Could you check a few things on this model? Use its own coordinates, in mm. A direction names the side the tool comes from. Round coordinates to 2 decimals unless told otherwise and drop trailing zeros. Order: outer loops, then holes, each group sorted by start corner. A loop starts at its lowest first (then second) coordinate and runs counter-clockwise, first axis right, second up. Notation, with made-up numbers: (27.5, 40) - (54.5, 40) arc R16 cw to (54.5, 54) - close; hole circle Ø5 at (-31, -13). An arc over 180 degrees is marked (long way). Use one line per item in the form item = value.
from build123d import *

# Parameters (mm, degrees)
F2_R             = 8.25
F3_DEPTH         = 3
F4_R             = 8.55
F5_DEPTH         = 17.2
F7_S5_R          = 8.25
F7_T6_DEPTH      = 14
F6_R             = 6.25
F8_DEPTH         = 4
F10_D            = 10.3
F10_DEPTH        = 25
F10_TIP          = 3.094432188
F11_R            = 0.5
F12_SIZE         = 0.5
F14_DEPTH        = 8
F14_COPIES_COUNT = 2


# Not quite as in the source:
# - a fillet or chamfer that OpenCascade refuses, or shapes differently, is made with other operations: its cross-section is extruded or revolved along the edge and cut away or added
# - a pattern or mirror of a feature is missing from the dataset's text; its kind, count and spacing are read off the source's solid


with BuildPart() as f1:
    # F0 (on Right) → F1 (revolve)
    with BuildSketch(Plane.YZ):
        Polygon((0, 25), (0, 0), (57.36, 0), (57.36, 8.9099957178), (9.6, 15.875), (9.6, 15.375), (8, 15.375), (8, 15.875), (8, 25), align=None)
    revolve(axis=Axis((0, 28.68, 0), (0, 1, 0)))

    # F2 (on face) → F3 (join)
    with BuildSketch(Plane(origin=(0, 57.36, 0), x_dir=(-1, 0, 0), z_dir=(0, 1, 0))):
        Circle(F2_R)
    extrude(amount=F3_DEPTH)

    # F4 (on face) → F5 (join)
    with BuildSketch(Plane(origin=(0, 60.36, 0), x_dir=(-1, 0, 0), z_dir=(0, 1, 0))):
        Circle(F4_R)
    extrude(amount=F5_DEPTH)

    # F7: chamfer of 0.5 x 1.8660254038 on 1 edges, made by hand


with BuildPart() as f7_tool2:
    # F7_s3 → F7_t4 (revolve)
    with BuildSketch(Plane.XY):
        Polygon((-8.55, 60.86), (-6.6839745962, 60.36), (-8.55, 60.36), align=None)
    revolve(axis=Axis((0, 60.36, 0), (0, 1, 0)))

    # F7_s5 → F7_t6 (cut, symmetric)
    with BuildSketch(Plane.XZ.offset(-60.6)):
        Circle(F7_S5_R)
    extrude(amount=F7_T6_DEPTH, both=True, mode=Mode.SUBTRACT)


with BuildPart() as f1_1:
    add(f1.part)

    # F7_t1: cut F7_tool2
    add(f7_tool2.part, mode=Mode.SUBTRACT)

    # F6 (on face) → F8 (cut)
    with BuildSketch(Plane(origin=(0, 77.56, 0), x_dir=(-1, 0, 0), z_dir=(0, 1, 0))):
        Circle(F6_R)
    extrude(amount=-F8_DEPTH, mode=Mode.SUBTRACT)

    # F10
    with Locations(Plane(origin=(0, 73.56, 0), x_dir=(-1, 0, 0), z_dir=(0, 1, 0))):
        with Locations((0, 0)):
            Hole(F10_D / 2, depth=F10_DEPTH)
            with Locations((0, 0, -(F10_DEPTH + F10_TIP / 2))):  # 118° drill point
                Cone(0, F10_D / 2, F10_TIP, mode=Mode.SUBTRACT)

    # F11
    f11_edges = [f1_1.edges().sort_by_distance(p)[0] for p in [
        (0, 8, -25),
        (0, 0, -25),
        (0, 4, 25),
    ]]
    fillet(f11_edges, radius=F11_R)

    # F12
    f12_edges = [f1_1.edges().sort_by_distance(p)[0] for p in [
        (8.55, 77.56, 0),
        (6.25, 77.56, 0),
        (5.15, 73.56, 0),
    ]]
    chamfer(f12_edges, length=F12_SIZE)

    # F13 (on face) → F14 (cut, through all)
    with BuildSketch(Plane.XZ):
        Polygon((-8.0518, 15.7346906059), (0, 15.8726696123), (8.0518, 16.0106486188), (8.0518, 25), (-8.0518, 25), align=None)
    f14 = extrude(amount=-F14_DEPTH, mode=Mode.SUBTRACT)

    # F14_copies: F14 ×2 about axis
    f14_copies_axis = Axis((0, 0, 0), (0, 1, 0))
    for i in range(1, F14_COPIES_COUNT):
        add(f14.rotate(f14_copies_axis, i * 360 / F14_COPIES_COUNT), mode=Mode.SUBTRACT)


solid = f1_1.part
Item 1: If we mould it in two halves opening along Z, with no side actions, what happens to faces 1 (the face through (11, 8, 11)), 2 (the face through (5, 73.56, -3)), 3 (the face through (-13.64, 8.789, 7.095))? For each: released by +Z, released by -Z, zero draft, split by the parting line, or undercut.
Found:
face_1 = zero draft
face_2 = undercut
face_3 = split by the parting line
Item 2: I need wall thicknesses on L1, parallel to Z at x = 0, y = 74.95; L2, parallel to Z at x = 0, y = 68.25; L3, parallel to X at y = 66, z = 2.5. Which ranges of each line are inside material? Lowest first, please.
Found:
L1 = -8.55 to -6.25, 6.25 to 8.55
L2 = -8.55 to -5.15, 5.15 to 8.55
L3 = -8.18 to -4.5, 4.5 to 8.18
Item 3: Imagine slicing it at D-D on y = 26. Please give me the cut outline in (x, z).
Found:
outline = circle Ø26.97 at (0, 0)
Item 4: Imagine slicing it at B-B on y = 67.5. Please give me the cut outline in (x, z).
Found:
outline = circle Ø17.1 at (0, 0); hole circle Ø10.3 at (0, 0)
Item 5: Imagine slicing it at A-A on y = 5. Please give me the cut outline in (x, z), plus the area to 3 significant figures.
Found:
outline = (-8.05, -23.67) - (-8.05, -16.01) - (8.05, -15.73) - (8.05, -23.67) arc R25 ccw to (8.05, 23.67) - (8.05, 16.01) - (-8.05, 15.73) - (-8.05, 23.67) arc R25 ccw to start
area = 1,680 mm2
Item 6: Will these pins go through, and if not, where does the flat tip stop? P1, Ø9.5, axis at x = 0, z = 0, coming from the +Y side; P2, Ø8, axis at y = 22.5, z = -4, coming from the -X side; P3, Ø4, axis at x = 4, y = 38.5, coming from the -Z side.
Found:
P1 = 48.32
P2 = -14.37
P3 = -11.59
Item 7: For faces 4 (the face through (8.052, 4, -20)), 5 (the face through (-8, 57.36, -3)), 6 (the face through (4.91, 60.64, 1.55)), 7 (the face through (8.052, 4, 20)), which set-ups out of +Z, -Z, +X, -X, +Y, -Y let a thin tool reach every point of the face, with its end or its side?
Found:
face_4 = -Z, +Y, -Y
face_5 = none
face_6 = +Y
face_7 = +Z, +Y, -Y
Item 8: Imagine slicing it at C-C on y = 18. Please give me the cut outline in (x, z).
Found:
outline = circle Ø29.3 at (0, 0)
